Design review of the part built by this model. Coordinates are the model's own, in mm. A direction names the side the tool comes from. Round coordinates to 2 decimals unless told otherwise and drop trailing zeros. Loops run counter-clockwise (first coordinate to the right, second up) from the corner with the lowest first, then second, coordinate; pieces in that order, holes last. Notation, with made-up numbers: M 67,39.25 L 106,39.25 A17 cw 106,49.25 Z; hole C 44,-6.5 d8. An arc over 180 degrees is marked long. Use a Markdown table: item, result.
from build123d import *

# Parameters (mm, degrees)
SKETCH_1_W          = 100
SKETCH_1_H          = 68
EXTRUDE_1_DEPTH     = 3
SKETCH_2_W          = 100
SKETCH_2_H          = 3
EXTRUDE_2_DEPTH     = 27
SKETCH_3_W          = 7
SKETCH_3_H          = 24
CUT_EXTRUDE_2_DEPTH = 27
SKETCH_4_W          = 62
SKETCH_4_H          = 5
EXTRUDE_3_DEPTH     = 52
SKETCH_5_R          = 1.5
CUT_EXTRUDE_4_DEPTH = 5
SKETCH_7_W          = 35
SKETCH_7_H          = 48
CUT_EXTRUDE_5_DEPTH = 3
SKETCH_8_W          = 55
SKETCH_8_H          = 3
EXTRUDE_4_DEPTH     = 45
SKETCH_11_W         = 55
SKETCH_11_H         = 3
EXTRUDE_5_DEPTH     = 45
SKETCH_10_R         = 2
SKETCH_10_W         = 32
SKETCH_10_H         = 36
CUT_EXTRUDE_6_DEPTH = 45
SKETCH_12_R         = 3
CUT_EXTRUDE_7_DEPTH = 2
SKETCH_13_W         = 40
SKETCH_13_H         = 27.004423226
CUT_EXTRUDE_8_DEPTH = 3
FILLET_1_R          = 20


with BuildPart() as part:
    # 스케치1 → 보스-돌출1 (new body)
    with BuildSketch(Plane(origin=(0, 0, 0), x_dir=(1, 0, 0), z_dir=(0, 1, 0))):
        Rectangle(SKETCH_1_W, SKETCH_1_H)
    extrude(amount=EXTRUDE_1_DEPTH)

    # 스케치2 → 보스-돌출2 (add)
    with BuildSketch(Plane(origin=(0, 3, 0), x_dir=(1, 0, 0), z_dir=(0, 1, 0))):
        with Locations((0, 32.5)):
            Rectangle(SKETCH_2_W, SKETCH_2_H)
    extrude(amount=EXTRUDE_2_DEPTH)

    # 스케치3 → 컷-돌출2 (cut)
    with BuildSketch(Plane.XY.offset(-31)):
        with Locations((-35, 15)):
            Rectangle(SKETCH_3_W, SKETCH_3_H)
        with Locations((35, 15)):
            Rectangle(SKETCH_3_W, SKETCH_3_H)
    extrude(amount=-CUT_EXTRUDE_2_DEPTH, mode=Mode.SUBTRACT)

    # 스케치4 → 보스-돌출3 (add)
    with BuildSketch(Plane(origin=(0, 3, 0), x_dir=(1, 0, 0), z_dir=(0, 1, 0))):
        with Locations((0, -31.5)):
            Rectangle(SKETCH_4_W, SKETCH_4_H)
    extrude(amount=EXTRUDE_3_DEPTH)

    # 스케치5 → 컷-돌출4 (cut)
    with BuildSketch(Plane.XY.offset(34)):
        with Locations((-23, 30)):
            Circle(SKETCH_5_R)
        with Locations((23, 30)):
            Circle(SKETCH_5_R)
        with BuildLine():
            Line((-15, 30), (-15, 3))
            Line((-15, 3), (15, 3))
            Line((15, 3), (15, 30))
            ThreePointArc((15, 30), (0, 45), (-15, 30))
        make_face()
    extrude(amount=-CUT_EXTRUDE_4_DEPTH, mode=Mode.SUBTRACT)

    # 스케치7 → 컷-돌출5 (cut)
    with BuildSketch(Plane.XZ):
        with Locations((22.5, 0)):
            Rectangle(SKETCH_7_W, SKETCH_7_H)
        with Locations((-22.5, 0)):
            Rectangle(SKETCH_7_W, SKETCH_7_H)
    extrude(amount=-CUT_EXTRUDE_5_DEPTH, mode=Mode.SUBTRACT)

    # 스케치8 → 보스-돌출4 (add)
    with BuildSketch(Plane(origin=(50, 0, 0), x_dir=(0, 0, -1), z_dir=(1, 0, 0))):
        with Locations((6.5, 1.5)):
            Rectangle(SKETCH_8_W, SKETCH_8_H)
    extrude(amount=EXTRUDE_4_DEPTH)

    # 스케치11 → 보스-돌출5 (add)
    with BuildSketch(Plane.ZY.offset(50)):
        with Locations((-6.5, 1.5)):
            Rectangle(SKETCH_11_W, SKETCH_11_H)
    extrude(amount=EXTRUDE_5_DEPTH)

    # 스케치10 → 컷-돌출6 (cut)
    with BuildSketch(Plane(origin=(0, 3, 0), x_dir=(1, 0, 0), z_dir=(0, 1, 0))):
        with Locations((55.5, -15.5)):
            Circle(SKETCH_10_R)
        with Locations((55.5, 28.5)):
            Circle(SKETCH_10_R)
        with Locations((89.5, 28.5)):
            Circle(SKETCH_10_R)
        with Locations((89.5, -15.5)):
            Circle(SKETCH_10_R)
        with Locations((-89.5, -15.5)):
            Circle(SKETCH_10_R)
        with Locations((-55.5, -15.5)):
            Circle(SKETCH_10_R)
        with Locations((-55.5, 28.5)):
            Circle(SKETCH_10_R)
        with Locations((-89.5, 28.5)):
            Circle(SKETCH_10_R)
        with Locations((72.5, 6.5)):
            Rectangle(SKETCH_10_W, SKETCH_10_H)
        with Locations((-72.5, 6.5)):
            Rectangle(SKETCH_10_W, SKETCH_10_H)
    extrude(amount=-CUT_EXTRUDE_6_DEPTH, mode=Mode.SUBTRACT)

    # 스케치12 → 컷-돌출7 (cut)
    with BuildSketch(Plane.XZ):
        with Locations((89.5, -28.5)):
            Circle(SKETCH_12_R)
        with Locations((89.5, 15.5)):
            Circle(SKETCH_12_R)
        with Locations((55.5, 15.5)):
            Circle(SKETCH_12_R)
        with Locations((55.5, -28.5)):
            Circle(SKETCH_12_R)
        with Locations((-89.5, 15.5)):
            Circle(SKETCH_12_R)
        with Locations((-55.5, 15.5)):
            Circle(SKETCH_12_R)
        with Locations((-55.5, -28.5)):
            Circle(SKETCH_12_R)
        with Locations((-89.5, -28.5)):
            Circle(SKETCH_12_R)
    extrude(amount=-CUT_EXTRUDE_7_DEPTH, mode=Mode.SUBTRACT)

    # 스케치13 → 컷-돌출8 (cut)
    with BuildSketch(Plane(origin=(0, 0, -34), x_dir=(-1, 0, 0), z_dir=(0, 0, -1))):
        with Locations((0, 16.497788387)):
            Rectangle(SKETCH_13_W, SKETCH_13_H)
    extrude(amount=-CUT_EXTRUDE_8_DEPTH, mode=Mode.SUBTRACT)

    # 필렛1
    fillet_1_edges = [part.edges().sort_by_distance(p)[0] for p in [
        (31, 55, 31.5),
        (-31, 55, 31.5),
    ]]
    fillet(fillet_1_edges, radius=FILLET_1_R)


solid = part.part
1. Machinability: for faces 4 (the face through (-31, 19, 32)), 5 (the face through (52.5, 1, 15.6)), 6 (the face through (-15, 17, 32)), 7 (the face through (-39, 16, -31)), which of the approach directions +Z, -Z, +X, -X, +Y, -Y give a long, thin tool a straight path to every point of the face, cutting with its end or side? Answer none if there is none.
Check values:
| item | result |
|---|---|
| face 4 | +Z, -X, +Y |
| face 5 | -Y |
| face 6 | +Z, -Z |
| face 7 | +X, -X, +Y |
2. Take a section at B-B on x = 64. Give the boundary of the cut face in (y, z).
Check values:
| item | result |
|---|---|
| outline | M 0,-34 L 3,-34 L 3,-24.5 L 0,-24.5 Z; M 0,11.5 L 3,11.5 L 3,21 L 0,21 Z |
3. Wall thickness on line 1 along Z through (x, y) = (-55.5, 2.8); line 2 along X through (y, z) = (2.4, -28.5); line 3 along Z through (x, y) = (89, 1): over which ranges is each line inside the solid? List them lowest first. Write a range as from..to.
Check values:
| item | result |
|---|---|
| line 1 | z = -34..-30.5, -26.5..13.5, 17.5..21 |
| line 2 | x = -95..-91.5, -87.5..-57.5, -53.5..53.5, 57.5..87.5, 91.5..95 |
| line 3 | z = -34..-31.46, -25.54..12.54, 18.46..21 |
4. The part is to be moulded in two halves that separate along X. For faces 1 (the face through (0, 46, 29)), 2 (the face through (-56, 2, 18)), 3 (the face through (-25.297, 48.986, 31.465)), say which applies: pulls with the +X half, pulls with the -X half, needs draft (parallel to the pull), parting line crosses it, or undercut.
Check values:
| item | result |
|---|---|
| face 1 | needs draft |
| face 2 | undercut |
| face 3 | pulls with the -X half |
5. Take a section at A-A on y = 13. Give the boundary of the cut face in (x, z), and give its area (3 significant figures).
Check values:
| item | result |
|---|---|
| outline | M -50,-34 L -38.5,-34 L -38.5,-31 L -50,-31 Z; M -31.5,-34 L -20,-34 L -20,-31 L -31.5,-31 Z; M -31,29 L -15,29 L -15,34 L -31,34 Z; M 15,29 L 31,29 L 31,34 L 15,34 Z; M 20,-34 L 31.5,-34 L 31.5,-31 L 20,-31 Z; M 38.5,-34 L 50,-34 L 50,-31 L 38.5,-31 Z |
| area | 298 mm² |
6. Take a section at D-D on y = 39.5. Give the boundary of the cut face in (x, z).
Check values:
| item | result |
|---|---|
| outline | M -30.49,29 L -11.61,29 L -11.61,34 L -30.49,34 Z; M 11.61,29 L 30.49,29 L 30.49,34 L 11.61,34 Z |
7. Insertion check: pin 1 (3.5 mm diameter, centred on y = 1.5, z = 28, fed in from +X); pin 2 (3.5 mm diameter, centred on x = -55.5, z = -28.5, fed in from -Y); pin 3 (1.5 mm diameter, centred on y = 16, z = 30.5, fed in from +X); pin 4 (0.9 mm diameter, centred on x = -41, z = -32, fed in from +Y). Each pin has a flat end and moves straight along its axis. Give the tip position at first contact, or say it passes through.
Check values:
| item | result |
|---|---|
| pin 1 | stops at x = 50 |
| pin 2 | passes through |
| pin 3 | stops at x = 31 |
| pin 4 | stops at y = 30 |
8. Take a section at C-C on z = -6. Give the boundary of the cut face in (x, y).
Check values:
| item | result |
|---|---|
| outline | M -95,0 L -88.5,0 L -88.5,3 L -95,3 Z; M -56.5,0 L -40,0 L -40,3 L -56.5,3 Z; M -5,0 L 5,0 L 5,3 L -5,3 Z; M 40,0 L 56.5,0 L 56.5,3 L 40,3 Z; M 88.5,0 L 95,0 L 95,3 L 88.5,3 Z |
